Autodesk Inventor part; units mm, degrees
ref_plane "YZ Plane" through (0, 0, 0) normal (1, 0, 0) x (0, 1, 0)
ref_plane "XZ Plane" through (0, 0, 0) normal (0, 1, 0) x (-1, 0, 0)
ref_plane "XY Plane" through (0, 0, 0) normal (0, 0, 1) x (1, 0, 0)
sketch "Sketch_1" plane through (0, 0, 0) normal (0, 0, 1) x (1, 0, 0)
  line L0 (85, 0) -> (-12, 0)
  line L1 (-12, 0) -> (-12, 2.75)
  line L2 (-12, 2.75) -> (-10.75, 4)
  line L3 (-10.75, 4) -> (-0.3, 4)
  arc A0 (-0.3, 4) -> (0, 4.3) centre (-0.3, 4.3) ccw
  line L4 (0, 4.3) -> (0, 5.5)
  line L5 (0, 5.5) -> (0.5, 6)
  line L6 (0.5, 6) -> (84.5, 6)
  line L7 (84.5, 6) -> (85, 5.5)
  line L8 (85, 5.5) -> (85, 0)
  line L9 (85, 0) -> (-12, 0)
revolve "Revolution1" add sketch "Sketch_1" angle 360 about axis through (85, 0, 0) along (1, 0, 0)
properties part number "SSFCU12-85-F12-P8"
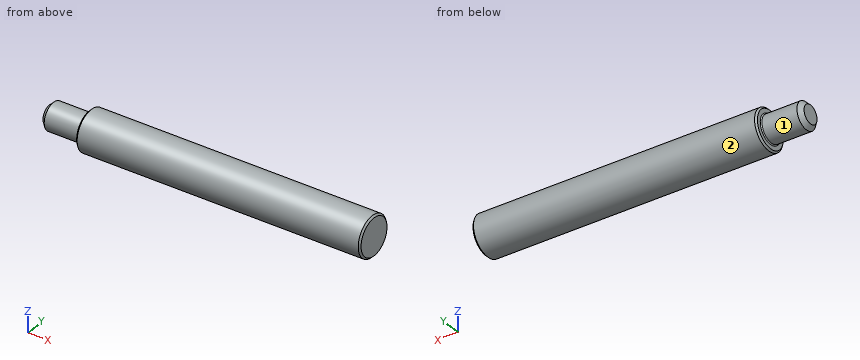
CAD build for the part. Positions are in the model's coordinates, mm. Face numbers are marked on the shaded views. A direction names the side the tool comes from. Coordinates: 2 decimals unless noted, no trailing zeros. Loops run counter-clockwise (first coordinate to the right, second up) from the corner with the lowest first, then second, coordinate; pieces in that order, holes last. Notation, with made-up numbers: (-37.5, -13.75) - (-7.5, -13.75) arc R21 cw to (-7.5, 12.25) - close; hole circle Ø1 at (42, 15.25). An arc over 180 degrees is marked (long way). Return JSON: item names as keys, results as strings.
1. Probe L1, parallel to Y at x = 79.5, z = 0.25; L2, parallel to X at y = 5, z = -1.5; L3, parallel to X at y = 2.5, z = -5. List the from-to ranges inside material, lowest first. Write a range as from..to.
Result:
{"L1": "y = -5.99..5.99", "L2": "x = 0..85", "L3": "x = 0.09..84.91"}
2. Drop flat-ended pins along their axis: pin 1 (1 mm diameter, centred on x = 24, y = 3.5, fed in from +Z); pin 2 (5 mm diameter, centred on x = 70.5, y = 4.5, fed in from -Z); pin 3 (5 mm diameter, centred on y = -4, z = -4.5, fed in from -X). Give the stop position or say it passes through.
Result:
{"pin 1": "stops at z = 5.2", "pin 2": "stops at z = -5.66", "pin 3": "stops at x = -11.23"}
3. Band-saw the part on A-A (z = 0). Give the cut face in (x, y).
Result:
{"outline": "(-12, -2.75) - (-10.75, -4) - (-0.3, -4) arc R0.3 cw to (0, -4.3) - (0, -5.5) - (0.5, -6) - (84.5, -6) - (85, -5.5) - (85, 5.5) - (84.5, 6) - (0.5, 6) - (0, 5.5) - (0, 4.3) arc R0.3 cw to (-0.3, 4) - (-10.75, 4) - (-12, 2.75) - close"}
4. 3-axis set-ups, long thin cutter, end or side, ignore diameter. For the marked faces 1 and 2: which of +Z, -Z, +X, -X, +Y, -Y reach the whole face in a straight line?
Result:
{"face 1": "-X", "face 2": "+X, -X"}
5. Band-saw the part on C-C (x = 30). Give the cut face in (y, z).
Result:
{"outline": "circle Ø12 at (0, 0)"}
